Model file for the job. Use its own axes, mm. Give positions to 0.01 mm unless a question says otherwise; leave off trailing zeros. Loops run counter-clockwise (first coordinate to the right, second up) from the corner with the lowest first, then second, coordinate; pieces in that order, holes last. Notation, with made-up numbers: (-5, 84) - (13, 84) arc R22 cw to (13, 95) - close; hole circle Ø10 at (59.25, 20.5). An arc over 180 degrees is marked (long way). Answer as CSV lines item,"result". Start each with the question number.
Item 1: Saw through at A-A on z = 25. Give the cut face in (x, y), plus the area to 3 significant figures.
Item 2: Drill centre lines: L1, parallel to X at y = 1.8, z = 25; L2, parallel to Z at x = 56, y = 1.3; L3, parallel to X at y = 0.6, z = 18. Where is each one in solid material? Low to high. Write a range as from..to.
Item 3: Saw through at C-C on y = 2.1. State how many separate pieces and enclosed holes the cut face has, plus the area to 3 significant figures.
Item 4: Pin check, flat tips, straight feed: pin 1 (1.2 mm diameter, centred on x = 76.55, z = 9.95, fed in from -Y); pin 2 (1.5 mm diameter, centred on y = 2, z = 17, fed in from -X); pin 3 (8 mm diameter, centred on x = 45.5, z = 7.5, fed in from -Y); pin 4 (0.9 mm diameter, centred on y = 2, z = 45.5, fed in from -X). Stop position of each tip, or through.
Item 5: Saw through at B-B on z = 33.5. Give the cut face in (x, y), plus the area to 3 significant figures.
Item 6: Saw through at D-D on z = 11.5. Give the cut face in (x, y), plus the area to 3 significant figures.
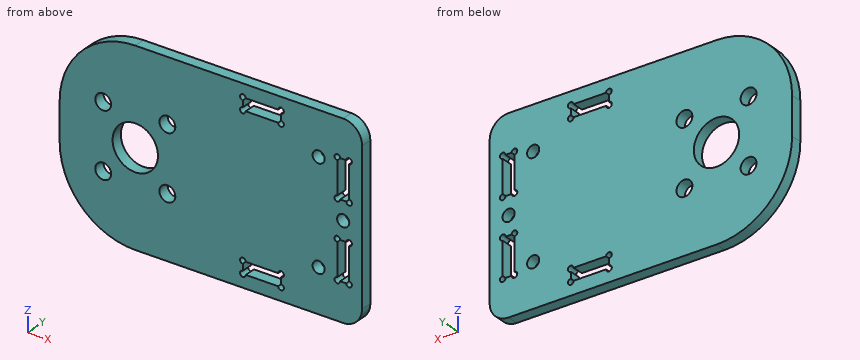
from build123d import *

# Parameters (mm, degrees)
SKETCH_1_W          = 80
SKETCH_1_H          = 50
EXTRUDE_1_DEPTH     = 3
SKETCH_2_R          = 6
SKETCH_2_R_2        = 2.1
CUT_EXTRUDE_1_DEPTH = 3
SKETCH_3_R          = 1.61
SKETCH_3_W          = 3.1
SKETCH_3_H          = 10.1
CUT_EXTRUDE_2_DEPTH = 3
SKETCH_4_R          = 1.6
SKETCH_4_W          = 10.1
SKETCH_4_H          = 3.2
CUT_EXTRUDE_3_DEPTH = 95.387499172
FILLET_1_R          = 20
FILLET_2_R          = 5
SKETCH_5_R          = 0.75
CUT_EXTRUDE_4_DEPTH = 95.387499172


with BuildPart() as part:
    # 草图1 → 凸台-拉伸1 (new body)
    with BuildSketch(Plane(origin=(0, 0, 0), x_dir=(1, 0, 0), z_dir=(0, 1, 0))):
        with Locations((40, -25)):
            Rectangle(SKETCH_1_W, SKETCH_1_H)
    extrude(amount=EXTRUDE_1_DEPTH)

    # 草图2 → 切除-拉伸1 (cut)
    with BuildSketch(Plane(origin=(0, 3, 0), x_dir=(1, 0, 0), z_dir=(0, 1, 0))):
        with Locations(Location((20, -25, 0), (0, 0, 270))):
            Circle(SKETCH_2_R)
        with Locations(Location((11.514718626, -16.514718626, 0), (0, 0, 270))):
            Circle(SKETCH_2_R_2)
        with Locations(Location((28.485281374, -16.514718626, 0), (0, 0, 270))):
            Circle(SKETCH_2_R_2)
        with Locations(Location((28.485281374, -33.485281374, 0), (0, 0, 270))):
            Circle(SKETCH_2_R_2)
        with Locations(Location((11.514718626, -33.485281374, 0), (0, 0, 270))):
            Circle(SKETCH_2_R_2)
    extrude(amount=-CUT_EXTRUDE_1_DEPTH, mode=Mode.SUBTRACT)

    # 草图3 → 切除-拉伸2 (cut)
    with BuildSketch(Plane(origin=(0, 3, 0), x_dir=(1, 0, 0), z_dir=(0, 1, 0))):
        with Locations(Location((75, -25, 0), (0, 0, 270))):
            Circle(SKETCH_3_R)
        with Locations((75, -15)):
            Rectangle(SKETCH_3_W, SKETCH_3_H)
        with Locations((75, -35)):
            Rectangle(SKETCH_3_W, SKETCH_3_H)
    extrude(amount=-CUT_EXTRUDE_2_DEPTH, mode=Mode.SUBTRACT)

    # 草图4 → 切除-拉伸3 (cut, through all)
    with BuildSketch(Plane(origin=(0, 3, 0), x_dir=(1, 0, 0), z_dir=(0, 1, 0))):
        with Locations(Location((68.5, -11.5, 0), (0, 0, 270))):
            Circle(SKETCH_4_R)
        with Locations(Location((68.5, -38.5, 0), (0, 0, 90))):
            Circle(SKETCH_4_R)
        with Locations((53.5, -5)):
            Rectangle(SKETCH_4_W, SKETCH_4_H)
        with Locations((53.5, -45)):
            Rectangle(SKETCH_4_W, SKETCH_4_H)
    extrude(amount=-CUT_EXTRUDE_3_DEPTH, mode=Mode.SUBTRACT)

    # 圆角1
    fillet_1_edges = [part.edges().sort_by_distance(p)[0] for p in [
        (0, 1.5, 0),
        (0, 1.5, 50),
    ]]
    fillet(fillet_1_edges, radius=FILLET_1_R)

    # 圆角2
    fillet_2_edges = [part.edges().sort_by_distance(p)[0] for p in [
        (80, 1.5, 0),
        (80, 1.5, 50),
    ]]
    fillet(fillet_2_edges, radius=FILLET_2_R)

    # 草图5 → 切除-拉伸4 (cut, through all)
    with BuildSketch(Plane(origin=(0, 3, 0), x_dir=(1, 0, 0), z_dir=(0, 1, 0))):
        with Locations((48.45, -3.4)):
            Circle(SKETCH_5_R)
        with Locations((48.45, -6.6)):
            Circle(SKETCH_5_R)
        with Locations((58.55, -6.6)):
            Circle(SKETCH_5_R)
        with Locations((58.55, -3.4)):
            Circle(SKETCH_5_R)
        with Locations((73.45, -9.95)):
            Circle(SKETCH_5_R)
        with Locations((76.55, -9.95)):
            Circle(SKETCH_5_R)
        with Locations((76.55, -20.05)):
            Circle(SKETCH_5_R)
        with Locations((73.45, -20.05)):
            Circle(SKETCH_5_R)
        with Locations((73.45, -29.95)):
            Circle(SKETCH_5_R)
        with Locations((76.55, -29.95)):
            Circle(SKETCH_5_R)
        with Locations((76.55, -40.05)):
            Circle(SKETCH_5_R)
        with Locations((73.45, -40.05)):
            Circle(SKETCH_5_R)
        with Locations((58.55, -46.6)):
            Circle(SKETCH_5_R)
        with Locations((58.55, -43.4)):
            Circle(SKETCH_5_R)
        with Locations((48.45, -43.4)):
            Circle(SKETCH_5_R)
        with Locations((48.45, -46.6)):
            Circle(SKETCH_5_R)
    extrude(amount=-CUT_EXTRUDE_4_DEPTH, mode=Mode.SUBTRACT)


solid = part.part
Responses:
1,outline,"(0, 0) - (14, 0) - (14, 3) - (0, 3) - close; (26, 0) - (73.39, 0) - (73.39, 3) - (26, 3) - close; (76.61, 0) - (80, 0) - (80, 3) - (76.61, 3) - close"
1,area,"194 mm2"
2,L1,"0..14, 26..73.39, 76.61..80"
2,L2,"0..3.4, 6.6..43.4, 46.6..50"
2,L3,"0.1..10.03, 13..27, 29.97..73.45, 76.55..80"
3,separate pieces,"1"
3,enclosed holes,"12"
3,area,"3,480 mm2"
4,pin 1,"through"
4,pin 2,"x = 0.13"
4,pin 3,"y = 0"
4,pin 4,"x = 6.83"
5,outline,"(0.31, 0) - (9.41, 0) - (9.41, 3) - (0.31, 3) - close; (13.61, 0) - (26.39, 0) - (26.39, 3) - (13.61, 3) - close; (30.59, 0) - (73.45, 0) - (73.45, 3) - (30.59, 3) - close; (76.55, 0) - (80, 0) - (80, 3) - (76.55, 3) - close"
5,area,"205 mm2"
6,outline,"(1.9, 0) - (66.9, 0) - (66.9, 3) - (1.9, 3) - close; (70.1, 0) - (73.45, 0) - (73.45, 3) - (70.1, 3) - close; (76.55, 0) - (80, 0) - (80, 3) - (76.55, 3) - close"
6,area,"215 mm2"
